Input: part model. Units: mm. Frame: model coordinates. Coordinates: 2 decimals unless noted, no trailing zeros. Write each loop counter-clockwise with the first axis right and the second up, starting at its lowest first coordinate (ties: lowest second). Pieces come first, ordered by that corner, then holes. Notation, with made-up numbers: (-6.5, 31) -> (31.5, 31) arc R17 cw to (31.5, 51) -> close; hole circle Ø2 at (26.25, 85.5). An arc over 180 degrees is marked (long way). One line per question, with ' | ' between items. Start each with the question number.
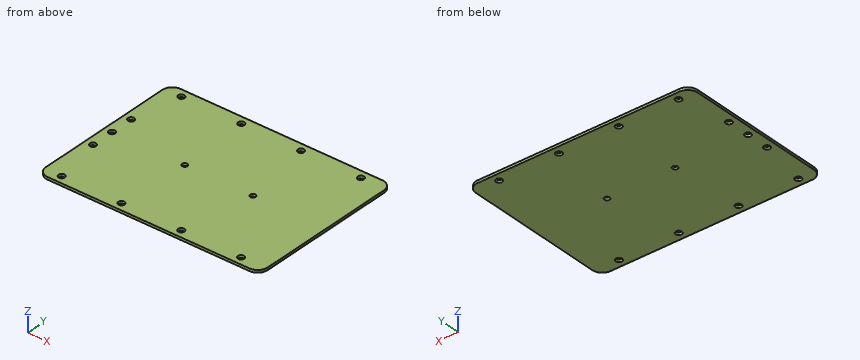
```python
from build123d import *

# Parameters (mm, degrees)
SKETCH1_W             = 133.501685986
SKETCH1_H             = 96.825
BOSS_EXTRUDE1_DEPTH   = 1.5
F_6_CLEARANCE_HOLE1_D = 3.7973
LPATTERN1_COUNT       = 4
LPATTERN1_PITCH       = 36
MIRROR1_COPY_1_D      = 3.7973
MIRROR1_COPY_2_D      = 3.7973
MIRROR1_COPY_3_D      = 3.7973
F_6_CLEARANCE_HOLE2_D = 3.7973
LPATTERN2_COUNT       = 3
LPATTERN2_PITCH       = 13.8875
FILLET1_R             = 6
SKETCH11_R            = 1.6
CUT_EXTRUDE1_DEPTH    = 112.42654106


with BuildPart() as part:
    # Sketch1 → Boss-Extrude1 (new body)
    with BuildSketch(Plane.XY):
        with Locations((2.475842993, -38.8875)):
            Rectangle(SKETCH1_W, SKETCH1_H)
    extrude(amount=BOSS_EXTRUDE1_DEPTH)

    # #6 Clearance Hole1 (through all)
    with Locations(Plane.XY.offset(1.5)):
        with Locations((54.226685986, 4.7625)):
            f_6_clearance_hole1 = Hole(F_6_CLEARANCE_HOLE1_D / 2)

    # LPattern1: #6 Clearance Hole1 ×4
    with Locations(*[(-i * LPATTERN1_PITCH, 0, 0) for i in range(1, LPATTERN1_COUNT)]):
        add(f_6_clearance_hole1, mode=Mode.SUBTRACT)

    # Mirror1: #6 Clearance Hole1 across plane
    add(f_6_clearance_hole1.mirror(Plane.ZX.offset(-38.8875)), mode=Mode.SUBTRACT)

    # Mirror1 copy 1 (through all)
    with Locations(Plane(origin=(-36, -77.775, 1.5), x_dir=(1, 0, 0), z_dir=(0, 0, 1))):
        with Locations((54.226685986, -4.7625)):
            Hole(MIRROR1_COPY_1_D / 2)

    # Mirror1 copy 2 (through all)
    with Locations(Plane(origin=(-72, -77.775, 1.5), x_dir=(1, 0, 0), z_dir=(0, 0, 1))):
        with Locations((54.226685986, -4.7625)):
            Hole(MIRROR1_COPY_2_D / 2)

    # Mirror1 copy 3 (through all)
    with Locations(Plane(origin=(-108, -77.775, 1.5), x_dir=(1, 0, 0), z_dir=(0, 0, 1))):
        with Locations((54.226685986, -4.7625)):
            Hole(MIRROR1_COPY_3_D / 2)

    # #6 Clearance Hole2 (through all)
    with Locations(Plane.XY.offset(1.5)):
        with Locations((-59.5125, -52.775)):
            f_6_clearance_hole2 = Hole(F_6_CLEARANCE_HOLE2_D / 2)

    # LPattern2: #6 Clearance Hole2 ×3
    with Locations(*[(0, i * LPATTERN2_PITCH, 0) for i in range(1, LPATTERN2_COUNT)]):
        add(f_6_clearance_hole2, mode=Mode.SUBTRACT)

    # Fillet1
    fillet1_edges = [part.edges().sort_by_distance(p)[0] for p in [
        (-64.275, -87.3, 0.75),
        (-64.275, 9.525, 0.75),
        (69.226685986, 9.525, 0.75),
        (69.226685986, -87.3, 0.75),
    ]]
    fillet(fillet1_edges, radius=FILLET1_R)

    # Sketch11 → Cut-Extrude1 (cut, through all)
    with BuildSketch(Plane(origin=(0, 0, 0), x_dir=(-1, 0, 0), z_dir=(0, 0, -1))):
        with Locations((-25.301031068, -38.88751017)):
            Circle(SKETCH11_R)
        with Locations((15.699384735, -38.887383169)):
            Circle(SKETCH11_R)
    extrude(amount=-CUT_EXTRUDE1_DEPTH, mode=Mode.SUBTRACT)


solid = part.part
```
1) Section A-A, the plane y = -25. Return loops of the section in (x, z) (3 decimals), then the cut area to 3 significant figures.
2) Ray query, line 1 (Y direction, x = 18.5, z = 0.65) (3 decimals); line 2 (Y direction, x = -19.5, z = 1.1) (3 decimals). Return the intervals inside material, ascending.
3) First-contact query: P1, Ø2.5, axis at x = -59.51, y = -52.78, coming from the -Z side. Flat tip, straight axial feed; report the tip coordinate or a pass-through.
Answer block:
1) outline: (-64.275, 0) -> (-61.411, 0) -> (-61.411, 1.5) -> (-64.275, 1.5) -> close; (-57.614, 0) -> (69.227, 0) -> (69.227, 1.5) -> (-57.614, 1.5) -> close | area: 195 mm2
2) line 1: y = -87.3 to -84.416, -80.659 to 2.884, 6.641 to 9.525 | line 2: y = -87.3 to -83.327, -81.748 to 3.973, 5.552 to 9.525
3) P1: passes through
